The listing builds one solid part. Answer for the finished solid, in the listing's coordinates (mm). A direction names the side the tool comes from. Coordinates: 2 decimals unless noted, no trailing zeros. Write each loop counter-clockwise with the first axis right and the second up, starting at its lowest first coordinate (ties: lowest second). Pieces come first, ordered by that corner, then holes.
(1) The part is cut by section D-D on x = 8.5. Determine the outline of the cut face in (y, z) (3 decimals), plus the area to 3 significant figures.
(2) Straight lines are drawn through the part: line 1 (Z direction, x = 1.5, y = 5); line 2 (Z direction, x = 8.75, y = 35); line 3 (Y direction, x = 6, z = -29.5). For each, find the intervals that lie inside material, in ascending order.
(3) The part is cut by section C-C on y = 41. Determine the outline of the cut face in (x, z), plus the area to 3 significant figures.
(4) Given P1, Ø1.5, axis at y = 26, z = -31, coming from the -X side; P2, Ø1.5, axis at x = 5, z = -9.5, coming from the +Y side; P3, Ø6, axis at x = 2.5, z = -33.5, coming from the -Y side; P4, Ø3, axis at x = 8.5, y = 34.5, coming from the +Z side, each flat-ended and moving along its own axis, determine where each tip first touches the part or whether it passes through.
(5) For a pull along Z with two mould halves and no side action, classify faces 1 (the cylindrical face through (6.26, 13.49, -35.81)), 2 (the flat face through (10, 32, -19.05)), 3 (the cylindrical face through (6.26, 4.6, -35.81)), 4 (the flat face through (0, 10, -22)) as +Z half, -Z half, draft (parallel to the pull), parting line (faces both ways), or undercut.
(6) Which of the six approach directions +Z, -Z, +X, -X, +Y, -Y give full straight-line access (tool end or side, diameter ignored) to faces 5 (the flat face through (6.858, 32, -32)), 6 (the flat face through (6, 9, 0))?
(7) The part is cut by section A-A on z = -40. Determine the outline of the cut face in (x, y).
(8) The part is cut by section B-B on x = 1. Determine the outline of the cut face in (y, z) (3 decimals).
from build123d import *

# Parameters (mm, degrees)
SKETCH1_W           = 44.45
SKETCH1_H           = 19.05
BOSS_EXTRUDE1_DEPTH = 12.7
SKETCH3_R           = 0.927000051
CUT_EXTRUDE1_DEPTH  = 50.99995
SKETCH4_W           = 5.842
SKETCH4_H           = 25.4
BOSS_EXTRUDE2_DEPTH = 25.654


with BuildPart() as part:
    # Sketch1 → Boss-Extrude1 (new body)
    with BuildSketch(Plane(origin=(0, 0, 0), x_dir=(0, 0, -1), z_dir=(1, 0, 0))):
        with Locations((22.225, 9.525)):
            Rectangle(SKETCH1_W, SKETCH1_H)
    extrude(amount=BOSS_EXTRUDE1_DEPTH)

    # Sketch3 → Cut-Extrude1 (cut, through all)
    with BuildSketch(Plane(origin=(0, 0, 0), x_dir=(0, 0, -1), z_dir=(1, 0, 0))):
        with Locations((9.525, 4.318)):
            Circle(SKETCH3_R)
        with Locations((34.925, 4.318)):
            Circle(SKETCH3_R)
        with Locations((34.925, 13.208)):
            Circle(SKETCH3_R)
        with Locations((9.525, 13.208)):
            Circle(SKETCH3_R)
    extrude(amount=CUT_EXTRUDE1_DEPTH, mode=Mode.SUBTRACT)

    # Sketch4 → Boss-Extrude2 (add)
    with BuildSketch(Plane(origin=(0, 19.05, 0), x_dir=(1, 0, 0), z_dir=(0, 1, 0))):
        with Locations((9.779, 31.75)):
            Rectangle(SKETCH4_W, SKETCH4_H)
    extrude(amount=BOSS_EXTRUDE2_DEPTH)


solid = part.part
Model answer:
1. outline: (0, -44.45) - (44.704, -44.45) - (44.704, -19.05) - (19.05, -19.05) - (19.05, 0) - (0, 0) - close; hole circle Ø1.854 at (4.318, -34.925); hole circle Ø1.854 at (4.318, -9.525); hole circle Ø1.854 at (13.208, -34.925); hole circle Ø1.854 at (13.208, -9.525)
1. area: 1,490 mm2
2. line 1: z = -44.45 to -35.55, -34.3 to -10.15, -8.9 to 0
2. line 2: z = -44.45 to -19.05
2. line 3: y = 0 to 19.05
3. outline: (6.86, -44.45) - (12.7, -44.45) - (12.7, -19.05) - (6.86, -19.05) - close
3. area: 148 mm2
4. P1: stops at x = 6.86
4. P2: stops at y = 19.05
4. P3: stops at y = 0
4. P4: stops at z = -19.05
5. face 1: undercut
5. face 2: +Z half
5. face 3: undercut
5. face 4: draft
6. face 5: +Z, -Z, -X, +Y
6. face 6: +Z, +X, -X, +Y, -Y
7. outline: (0, 0) - (12.7, 0) - (12.7, 44.7) - (6.86, 44.7) - (6.86, 19.05) - (0, 19.05) - close
8. outline: (0, -44.45) - (19.05, -44.45) - (19.05, 0) - (0, 0) - close; hole circle Ø1.854 at (4.318, -34.925); hole circle Ø1.854 at (4.318, -9.525); hole circle Ø1.854 at (13.208, -34.925); hole circle Ø1.854 at (13.208, -9.525)
